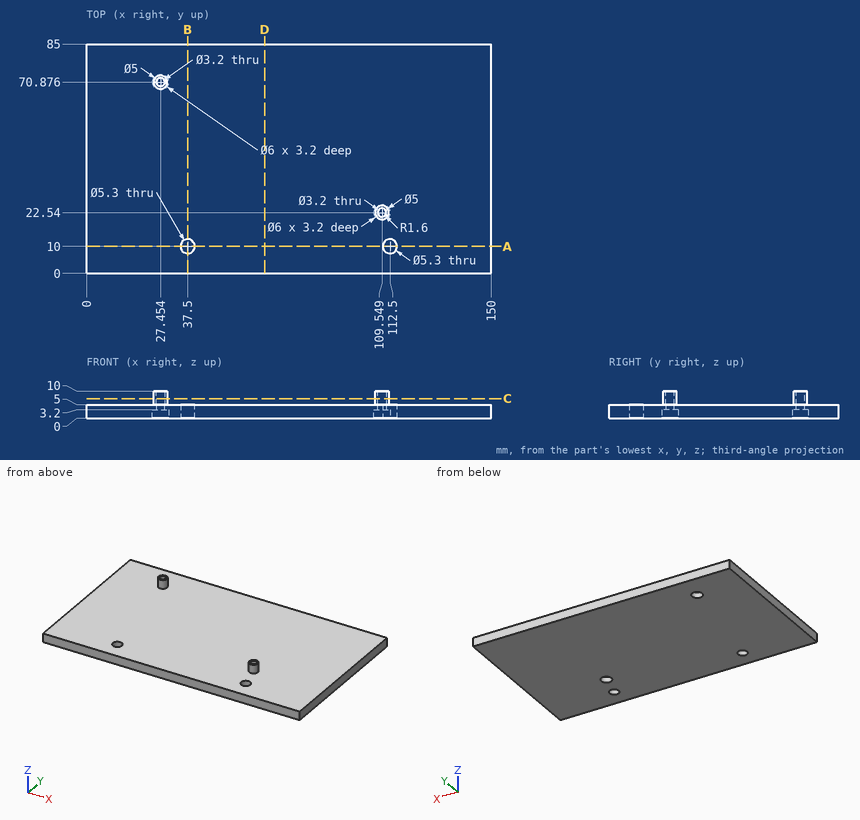
Geometry check sheet. Reference: drawing and pictorial views, mm from the part's lowest x, y, z. Round coordinates to 2 decimals unless told otherwise and drop trailing zeros. Loops run counter-clockwise (first coordinate to the right, second up) from the corner with the lowest first, then second, coordinate; pieces in that order, holes last. Notation, with made-up numbers: M 58.5,64 L 89.5,64 A14 ccw 89.5,91 Z; hole C 12,34 d5. An arc over 180 degrees is marked long. One line per item, written item: value.
(1) Sectioned sample at C-C, the plane z = 7.25. Count the separate pieces of the cut face and the enclosed holes in it.
Computed values:
separate pieces: 2
enclosed holes: 2
(2) Thickness scan on line 1 (Z direction, x = 132, y = 9); line 2 (Y direction, x = 109, z = 4); line 3 (Z direction, x = 111.5, y = 24.5). Record the ranges inside material, lowest first.
Computed values:
line 1: z = 0 to 5
line 2: y = 0 to 21.04, 24.04 to 85
line 3: z = 3.2 to 5
(3) Depth check by flat-ended pin: pin 1 Ø6 at (x, y) = (123, 26) entering from +Z; pin 2 Ø5 at (x, y) = (27.45, 70.88) entering from -Z. Enter the tip coordinate at first touch or a pass-through.
Computed values:
pin 1: stops at z = 5
pin 2: stops at z = 3.2
(4) Sectioned sample at D-D, the plane x = 66. Record the cut outline in (y, z).
Computed values:
outline: M 0,0 L 85,0 L 85,5 L 0,5 Z
(5) Sectioned sample at A-A, the plane y = 10. Record the cut outline in (x, z).
Computed values:
outline: M 0,0 L 34.85,0 L 34.85,5 L 0,5 Z; M 40.15,0 L 109.85,0 L 109.85,5 L 40.15,5 Z; M 115.15,0 L 150,0 L 150,5 L 115.15,5 Z
(6) Sectioned sample at B-B, the plane x = 37.5. Record the cut outline in (y, z).
Computed values:
outline: M 0,0 L 7.35,0 L 7.35,5 L 0,5 Z; M 12.65,0 L 85,0 L 85,5 L 12.65,5 Z
